Autodesk Inventor part; units mm, degrees
ref_plane "YZ Plane" through (0, 0, 0) normal (1, 0, 0) x (0, 1, 0)
ref_plane "XZ Plane" through (0, 0, 0) normal (0, 1, 0) x (-1, 0, 0)
ref_plane "XY Plane" through (0, 0, 0) normal (0, 0, 1) x (1, 0, 0)
sketch "Sketch1" plane through (0, 0, 0) normal (0, 1, 0) x (-1, 0, 0)
  circle A0 centre (0, 0) radius 12.7
  dimension "d0" = 25.4
extrude "Extrusion1" add sketch "Sketch1" along normal blind 151.2316
sketch "Sketch3" plane through (0, 151.2316, 0) normal (0, 1, 0) x (1, 0, 0)
  circle A0 centre (0, 0) radius 6.35
  dimension "d11" = 12.7
sketch "Sketch2" plane through (0, 0, 0) normal (0, -1, 0) x (1, 0, 0)
  circle A0 centre (0, 0) radius 3.175
  dimension "d3" = 6.35
hole "Hole1" at (0, 0, 0) direction (0, 1, 0) diameter 4.9784 depth 19.05 tip angle 118
hole "Hole2" at (0, 151.2316, 0) direction (0, -1, 0) diameter 4.9784 depth 19.05 tip angle 118
properties part number "feet type 1 part 2" material "Fiber Glass"
Input: part model. Units: mm. Frame: model coordinates. A direction names the side the tool comes from. Coordinates: 2 decimals unless noted, no trailing zeros. Loops run counter-clockwise (first coordinate to the right, second up) from the corner with the lowest first, then second, coordinate; pieces in that order, holes last. Notation, with made-up numbers: M 2,-20.5 L 40,-20.5 A5 cw 40,-13.5 Z; hole C 22,-20 d4. An arc over 180 degrees is marked long. Use a Markdown table: item, result. Add a question column.
1) Draft query along Z for faces 1 (the conical face through (-0.166, 20.286, -0.399)), 2 (the cylindrical face through (2.75, 74.56, 12.4)), 3 (the cylindrical face through (-0.748, 141.573, 2.374)), 4 (the flat face through (-3, 0, 0)). Return one class per face: +Z half, -Z half, draft (parallel to the pull), parting line (faces both ways), or undercut.
2) Pin query (flat end, axial travel): P1, Ø8, axis at y = 93, z = -3.5, coming from the +X side; P2, Ø8, axis at y = 80, z = -8, coming from the +X side; P3, Ø5, axis at x = -6, y = 58, coming from the -Z side; P4, Ø2, axis at x = -1.5, y = 45, coming from the +Z side. Return the tip coordinate at first contact, or that it passes through.
3) Line query: L1, parallel to Z at x = 0, y = 139.75; L2, parallel to X at y = 81, z = 0.5; L3, parallel to X at y = 94.5, z = -10.5. Output: solid intervals per line, ascending. Write a range as from..to.
4) Section B-B, the plane x = -9.5. Return the cut outline in (y, z), plus the area to 3 significant figures.
5) Set-up query: faces 5 (the conical face through (-0.422, 130.946, -0.094)), 6 (the cylindrical face through (-0.748, 9.658, -2.374)). Return all of +Z, -Z, +X, -X, +Y, -Y with unobstructed straight access to the full face (end or side cutting, diameter ignored); none if empty.
6) Section A-A, the plane z = 6.25. Return the cut outline in (x, y).
Answer below:
| question | item | result |
|---|---|---|
| 1 | face 1 | undercut |
| 1 | face 2 | parting line |
| 1 | face 3 | undercut |
| 1 | face 4 | draft |
| 2 | P1 | x = 12.7 |
| 2 | P2 | x = 12.05 |
| 2 | P3 | z = -12.21 |
| 2 | P4 | z = 12.69 |
| 3 | L1 | -12.7..-2.49, 2.49..12.7 |
| 3 | L2 | -12.69..12.69 |
| 3 | L3 | -7.14..7.14 |
| 4 | outline | M 0,-8.43 L 151.23,-8.43 L 151.23,8.43 L 0,8.43 Z |
| 4 | area | 2,550 mm2 |
| 5 | face 5 | +Y |
| 5 | face 6 | -Y |
| 6 | outline | M -11.06,0 L 11.06,0 L 11.06,151.23 L -11.06,151.23 Z |
